from build123d import *

# Parameters (mm, degrees)
SKETCH_1_W          = 50
SKETCH_1_H          = 49
EXTRUDE_1_DEPTH     = 4
SKETCH_2_R          = 2.5
CUT_EXTRUDE_1_DEPTH = 2
SKETCH_3_R          = 1.75
CUT_EXTRUDE_2_DEPTH = 4


with BuildPart() as part:
    # 草图1 → 凸台-拉伸1 (new body)
    with BuildSketch(Plane.XY):
        Rectangle(SKETCH_1_W, SKETCH_1_H)
    extrude(amount=EXTRUDE_1_DEPTH)

    # 草图2 → 切除-拉伸1 (cut)
    with BuildSketch(Plane.XY.offset(4)):
        with Locations((17.5, 17)):
            Circle(SKETCH_2_R)
        with Locations((-17.5, -17)):
            Circle(SKETCH_2_R)
    extrude(amount=-CUT_EXTRUDE_1_DEPTH, mode=Mode.SUBTRACT)

    # 草图3 → 切除-拉伸2 (cut)
    with BuildSketch(Plane.XY.offset(2)):
        with Locations((-17.5, -17)):
            Circle(SKETCH_3_R)
        with Locations((17.5, 17)):
            Circle(SKETCH_3_R)
    extrude(amount=-CUT_EXTRUDE_2_DEPTH, mode=Mode.SUBTRACT)


solid = part.part
The listing builds one solid part. Answer for the finished solid, in the listing's coordinates (mm). A direction names the side the tool comes from. Round coordinates to 2 decimals unless told otherwise and drop trailing zeros. Order: outer loops, then holes, each group sorted by start corner. A loop starts at its lowest first (then second) coordinate and runs counter-clockwise, first axis right, second up. Notation, with made-up numbers: M -5.75,34 L 49.25,34 A27 cw 49.25,73 Z; hole C 80,20 d1. An arc over 180 degrees is marked long. Answer in a Markdown table with one row per item. Add a question column.
1) The part is cut by section B-B on x = 17.5. Determine the outline of the cut face in (y, z).
2) Consider line 1 along Y through (x, z) = (-17.5, 3); line 2 along Y through (x, z) = (17.5, 3.1); line 3 along X through (y, z) = (-16, 0.65). Determine where each line is inside the solid, lowest interval first. Write a range as from..to.
3) Flat-ended cylindrical pins translate along their axes: pin 1 Ø4 at (x, y) = (-16.5, -17) entering from +Z; pin 2 Ø3 at (x, y) = (17.5, 17) entering from +Z; pin 3 Ø4 at (x, y) = (-17.5, -17) entering from +Z. Find the tip coordinate at first contact, or state that the pin passes through.
4) Which of the six approach directions +Z, -Z, +X, -X, +Y, -Y give full straight-line access (tool end or side, diameter ignored) to faces 1 (the face through (0, 0, 4)), 2 (the face through (-20, -17, 3))?
5) The part is cut by section A-A on y = -17. Determine the outline of the cut face in (x, z).
6) Determine the mould class of faces 3 (the face through (15, 17, 3)), 4 (the face through (0, -24.5, 2)), 5 (the face through (25, 0, 2)) for opening direction X: pulls with the +X half, pulls with the -X half, needs draft (parallel to the pull), parting line crosses it, or undercut.
7) The part is cut by section C-C on z = 2.9. Determine the outline of the cut face in (x, y), plus the area to 3 significant figures.
Findings below:
| question | item | result |
|---|---|---|
| 1 | outline | M -24.5,0 L 15.25,0 L 15.25,2 L 14.5,2 L 14.5,4 L -24.5,4 Z; M 18.75,0 L 24.5,0 L 24.5,4 L 19.5,4 L 19.5,2 L 18.75,2 Z |
| 2 | line 1 | y = -24.5..-19.5, -14.5..24.5 |
| 2 | line 2 | y = -24.5..14.5, 19.5..24.5 |
| 2 | line 3 | x = -25..-18.94, -16.06..25 |
| 3 | pin 1 | stops at z = 4 |
| 3 | pin 2 | passes through |
| 3 | pin 3 | stops at z = 2 |
| 4 | face 1 | +Z, +X, -X, +Y, -Y |
| 4 | face 2 | +Z |
| 5 | outline | M -25,0 L -19.25,0 L -19.25,2 L -20,2 L -20,4 L -25,4 Z; M -15.75,0 L 25,0 L 25,4 L -15,4 L -15,2 L -15.75,2 Z |
| 6 | face 3 | undercut |
| 6 | face 4 | needs draft |
| 6 | face 5 | pulls with the +X half |
| 7 | outline | M -25,-24.5 L 25,-24.5 L 25,24.5 L -25,24.5 Z; hole C -17.5,-17 d5; hole C 17.5,17 d5 |
| 7 | area | 2,410 mm² |
